from build123d import *

# Parameters (mm, degrees)
SKETCH1_W               = 74
SKETCH1_H               = 90
SKETCH1_R               = 2.6
BOSS_EXTRUDE1_DEPTH     = 10
SKETCH2_W               = 6
SKETCH2_H               = 90
BOSS_EXTRUDE2_DEPTH     = 69.85
SKETCH4_W               = 68
SKETCH4_H               = 25
CUT_EXTRUDE3_DEPTH      = 136.849263892
FILLET2_R               = 25
SKETCH8_W               = 29.83
SKETCH8_H               = 20
BOSS_EXTRUDE4_DEPTH     = 26
SKETCH9_R               = 6.75
CUT_EXTRUDE6_DEPTH      = 10
CUT_EXTRUDE7_START      = -10
SKETCH10_R              = 6.75
CUT_EXTRUDE7_DEPTH      = 10
SKETCH11_R              = 6.35
CUT_EXTRUDE8_DEPTH      = 4.9784
SKETCH12_W              = 25
SKETCH12_H              = 20
BOSS_EXTRUDE5_DEPTH     = 5
CUT_EXTRUDE9_DEPTH      = 134.202866961
CUT_EXTRUDE9_DEPTH_BACK = 134.202866961
SKETCH13_R              = 2.55
SKETCH14_R              = 2.6
CUT_EXTRUDE10_DEPTH     = 136.849263892


with BuildPart() as part:
    # Sketch1 → Boss-Extrude1 (new body)
    with BuildSketch(Plane.XY):
        with Locations((37, 45)):
            Rectangle(SKETCH1_W, SKETCH1_H)
        with Locations((50, 55)):
            Circle(SKETCH1_R, mode=Mode.SUBTRACT)
        with Locations((50, 35)):
            Circle(SKETCH1_R, mode=Mode.SUBTRACT)
    extrude(amount=BOSS_EXTRUDE1_DEPTH)

    # Sketch2 → Boss-Extrude2 (add)
    with BuildSketch(Plane(origin=(0, 0, 0), x_dir=(-1, 0, 0), z_dir=(0, 0, -1))):
        with Locations((-3, 45)):
            Rectangle(SKETCH2_W, SKETCH2_H)
    extrude(amount=BOSS_EXTRUDE2_DEPTH)

    # Sketch4 → Cut-Extrude3 (cut, through all)
    with BuildSketch(Plane(origin=(0, 0, 0), x_dir=(-1, 0, 0), z_dir=(0, 0, -1))):
        with Locations((-40, 77.5)):
            Rectangle(SKETCH4_W, SKETCH4_H)
        with Locations((-40, 12.5)):
            Rectangle(SKETCH4_W, SKETCH4_H)
    extrude(amount=-CUT_EXTRUDE3_DEPTH, mode=Mode.SUBTRACT)

    # Fillet2
    fillet2_edges = [part.edges().sort_by_distance(p)[0] for p in [
        (6, 65, 5),
        (6, 25, 5),
    ]]
    fillet(fillet2_edges, radius=FILLET2_R - 0.0001)  # a hair under: the kernel refuses the full size

    # Sketch8 → Boss-Extrude4 (add)
    with BuildSketch(Plane.ZY):
        with Locations((-4.915, 10)):
            Rectangle(SKETCH8_W, SKETCH8_H)
        with Locations((-4.915, 80)):
            Rectangle(SKETCH8_W, SKETCH8_H)
    extrude(amount=BOSS_EXTRUDE4_DEPTH)

    # Sketch9 → Cut-Extrude6 (cut)
    with BuildSketch(Plane.XZ):
        with Locations(Location((-16, -9.83, 0), (0, 0, 270))):
            Circle(SKETCH9_R)
    extrude(amount=-CUT_EXTRUDE6_DEPTH, mode=Mode.SUBTRACT)

    # Sketch10 → Cut-Extrude7 (cut)
    with BuildSketch(Plane(origin=(0, 90, 0), x_dir=(1, 0, 0), z_dir=(0, 1, 0)).offset(CUT_EXTRUDE7_START)):
        with Locations(Location((-16, 9.83, 0), (0, 0, 90))):
            Circle(SKETCH10_R)
    extrude(amount=CUT_EXTRUDE7_DEPTH, mode=Mode.SUBTRACT)

    # Sketch11 → Cut-Extrude8 (cut)
    with BuildSketch(Plane.ZY):
        with Locations((-53.5, 45)):
            Circle(SKETCH11_R)
    extrude(amount=-CUT_EXTRUDE8_DEPTH, mode=Mode.SUBTRACT)

    # Sketch12 → Boss-Extrude5 (add)
    with BuildSketch(Plane(origin=(6, 0, 0), x_dir=(0, 0, -1), z_dir=(1, 0, 0))):
        with Locations((57.35, 45)):
            Rectangle(SKETCH12_W, SKETCH12_H)
    extrude(amount=BOSS_EXTRUDE5_DEPTH)

    # Sketch13 → Cut-Extrude9 (cut, two sides: drawn at the far end of the back side and taken through both)
    with BuildSketch(Plane.ZY.offset(-4.9784).offset(-CUT_EXTRUDE9_DEPTH_BACK)):
        with Locations((-53.5, 45)):
            Circle(SKETCH13_R)
    extrude(amount=CUT_EXTRUDE9_DEPTH + CUT_EXTRUDE9_DEPTH_BACK, mode=Mode.SUBTRACT)

    # Sketch14 → Cut-Extrude10 (cut, through all)
    with BuildSketch(Plane.ZY):
        with Locations((-35, 70)):
            Circle(SKETCH14_R)
        with Locations((-35, 20)):
            Circle(SKETCH14_R)
        with Locations((-60.4, 70)):
            Circle(SKETCH14_R)
        with Locations((-60.4, 20)):
            Circle(SKETCH14_R)
    extrude(amount=-CUT_EXTRUDE10_DEPTH, mode=Mode.SUBTRACT)


solid = part.part
Part model, mm, in its own coordinate system. A direction names the side the tool comes from. Give positions to 0.01 mm unless a question says otherwise; leave off trailing zeros. Loops run counter-clockwise (first coordinate to the right, second up) from the corner with the lowest first, then second, coordinate; pieces in that order, holes last.
(1) Band-saw the part on A-A (z = -53.5). Write the cut outline in (x, y).
Return value:
outline: (0, 0) - (6, 0) - (6, 35) - (11, 35) - (11, 42.45) - (4.98, 42.45) - (4.98, 38.65) - (0, 38.65) - close; (0, 51.35) - (4.98, 51.35) - (4.98, 47.55) - (11, 47.55) - (11, 55) - (6, 55) - (6, 90) - (0, 90) - close
(2) Pin check, flat tips, straight feed: pin 1 (6.5 mm diameter, centred on x = -15, z = -7, fed in from -Y); pin 2 (8 mm diameter, centred on x = -7, z = -39, fed in from -Y); pin 3 (6 mm diameter, centred on x = 40, z = -2, fed in from +Y); pin 4 (1 mm diameter, centred on y = 46, z = -17.5, fed in from -X). Stop position of each tip, or through.
Return value:
pin 1: stops at y = 10
pin 2: passes through
pin 3: stops at y = 65
pin 4: stops at x = 0
(3) Band-saw the part on B-B (y = 45). Write the cut outline in (x, z).
Return value:
outline: (0, -69.85) - (11, -69.85) - (11, -56.05) - (4.98, -56.05) - (4.98, -59.85) - (0, -59.85) - close; (0, -47.15) - (4.98, -47.15) - (4.98, -50.95) - (11, -50.95) - (11, -44.85) - (6, -44.85) - (6, 0) - (74, 0) - (74, 10) - (0, 10) - close
(4) Band-saw the part on C-C (x = 3). Write the cut outline in (y, z).
Return value:
outline: (0, -69.85) - (90, -69.85) - (90, 10) - (0, 10) - close; hole circle Ø5.2 at (20, -60.4); hole circle Ø5.2 at (20, -35); hole circle Ø12.7 at (45, -53.5); hole circle Ø5.2 at (70, -60.4); hole circle Ø5.2 at (70, -35)
(5) 3-axis set-ups, long thin cutter, end or side, ignore diameter. For faces 1 (the cylindrical face through (-15.703, 4.93, -3.087)), 2 (the flat face through (8, 35, -57)), 3 (the cylindrical face through (-11.893, 84.93, -4.473)), 4 (the flat face through (4.978, 45.1, -50.8)), 5 (the flat face through (-13, 70, -5)): which of +Z, -Z, +X, -X, +Y, -Y reach the whole face in a straight line?
Return value:
face 1: -Y
face 2: -Z, +X, -Y
face 3: +Y
face 4: -X
face 5: +Z, -Z, -X
(6) Band-saw the part on D-D (z = -9.83). Write the cut outline in (x, y).
Return value:
outline: (-26, 0) - (-22.75, 0) - (-22.75, 10) - (-9.25, 10) - (-9.25, 0) - (6, 0) - (6, 90) - (-9.25, 90) - (-9.25, 80) - (-22.75, 80) - (-22.75, 90) - (-26, 90) - (-26, 70) - (0, 70) - (0, 20) - (-26, 20) - close
(7) Pull direction Z, two halves, no side cores. Call faces 6 (the flat face through (53, 25, 5)), 7 (the flat face through (4, 46, -69.85)), 8 (the flat face through (8, 45, -44.85)): pulls with the +Z half, pulls with the -Z half, needs draft (parallel to the pull), parting line crosses it, or undercut.
Return value:
face 6: needs draft
face 7: pulls with the -Z half
face 8: undercut
(8) Drill centre lines: line 1 along Y through (x, z) = (4.3, -35); line 2 along Z through (x, y) = (9, 45); line 3 along Y through (x, z) = (3, -53). Where is each one in solid material? Low to high.
Return value:
line 1: y = 0 to 17.4, 22.6 to 67.4, 72.6 to 90
line 2: z = -69.85 to -56.05, -50.95 to -44.85, 0 to 10
line 3: y = 0 to 38.67, 51.33 to 90
